```python
from build123d import *

# Parameters (mm, degrees)
SKETCH_1_R      = 1.75
SKETCH_1_W      = 12
SKETCH_1_H      = 4.5
EXTRUDE_1_DEPTH = 4.5
FILLET_1_R      = 12


with BuildPart() as part:
    # 草图1 → 凸台-拉伸1 (new body)
    with BuildSketch(Plane(origin=(0, 0, 0), x_dir=(1, 0, 0), z_dir=(0, 1, 0))):
        Polygon((29.444863729, 0), (14.722431864, 25.5), (-14.722431864, 25.5), (-29.444863729, 0), (-14.722431864, -25.5), (14.722431864, -25.5), align=None)
        Circle(SKETCH_1_R, mode=Mode.SUBTRACT)
        Polygon((13.887495374, 14.946152423), (9.990381057, 12.696152423), (15.990381057, 2.303847577), (19.887495374, 4.553847577), align=None, mode=Mode.SUBTRACT)
        with Locations((0, 17.25)):
            Rectangle(SKETCH_1_W, SKETCH_1_H, mode=Mode.SUBTRACT)
        Polygon((19.887495374, -4.553847577), (15.990381057, -2.303847577), (9.990381057, -12.696152423), (13.887495374, -14.946152423), align=None, mode=Mode.SUBTRACT)
        with Locations((0, -17.25)):
            Rectangle(SKETCH_1_W, SKETCH_1_H, mode=Mode.SUBTRACT)
        Polygon((-13.887495374, -14.946152423), (-9.990381057, -12.696152423), (-15.990381057, -2.303847577), (-19.887495374, -4.553847577), align=None, mode=Mode.SUBTRACT)
        Polygon((-19.887495374, 4.553847577), (-15.990381057, 2.303847577), (-9.990381057, 12.696152423), (-13.887495374, 14.946152423), align=None, mode=Mode.SUBTRACT)
    extrude(amount=EXTRUDE_1_DEPTH)

    # 圆角1
    fillet_1_edges = [part.edges().sort_by_distance(p)[0] for p in [
        (14.722431864, 2.25, 25.5),
        (-14.722431864, 2.25, 25.5),
        (-29.444863729, 2.25, 0),
        (-14.722431864, 2.25, -25.5),
        (14.722431864, 2.25, -25.5),
        (29.444863729, 2.25, 0),
    ]]
    fillet(fillet_1_edges, radius=FILLET_1_R)


solid = part.part
```
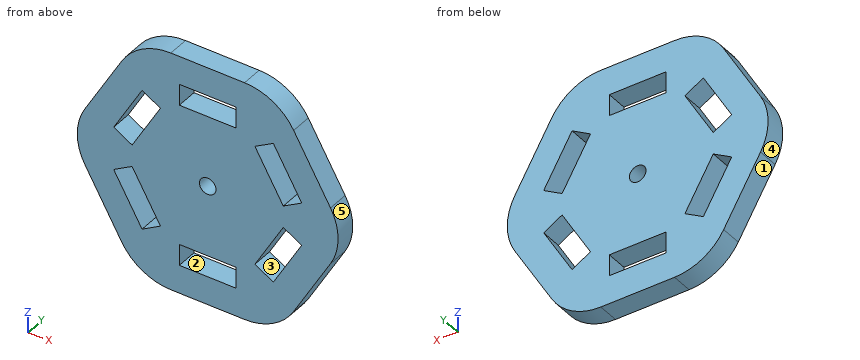
Check sheet for the modelled part. Datum: model origin and axes. Units: mm. Face numbers are marked on the shaded views. A direction names the side the tool comes from. Round coordinates to 2 decimals unless told otherwise and drop trailing zeros. Loops run counter-clockwise (first coordinate to the right, second up) from the corner with the lowest first, then second, coordinate; pieces in that order, holes last. Notation, with made-up numbers: (52.25, -13) - (111.25, -13) arc R23 cw to (111.25, 21) - close; hole circle Ø9 at (68.5, 69.25). An arc over 180 degrees is marked (long way). Write item = value, one per line. Start each with the question number.
Q1. Depth check by flat-ended pin: P1, Ø2, axis at y = 2.5, z = -16.5, coming from the -X side; P2, Ø3, axis at x = 0, z = 0, coming from the +Y side; P3, Ø2, axis at x = 20, y = 3, coming from the -Z side. Enter the tip coordinate at first touch or a pass-through.
Q2. Section check A-A (z = 0). Record the boundary of the cut face in (x, y).
Q3. Section check D-D (x = 15). Record the boundary of the cut face in (y, z).
Q4. Section check B-B (x = 0). Record the boundary of the cut face in (y, z).
Q5. Release check for a two-part mould opening along X. For the marked faces 3, 4 and 5 record: pulls with the +X half, pulls with the -X half, needs draft (parallel to the pull), parting line crosses it, or undercut.
Q6. Thickness scan on L1, parallel to Z at x = 0, y = 1.4; L2, parallel to Z at x = 4.5, y = 0.6; L3, parallel to X at y = 3.3, z = 0. Record the ranges inside material, lowest first.
Q7. Access from +Z, -Z, +X, -X, +Y, -Y to the whole of each face (thin tool, end or side, straight path). Record for the marked faces 1 and 2.
Q8. Section check C-C (z = 11). Record the boundary of the cut face in (x, y), plus the area to 3 significant figures.
Derived:
q1.P1 = -20.5
q1.P2 = through
q1.P3 = -18.09
q2.outline = (-27.59, 0) - (-1.75, 0) - (-1.75, 4.5) - (-27.59, 4.5) - close; (1.75, 0) - (27.59, 0) - (27.59, 4.5) - (1.75, 4.5) - close
q3.outline = (0, -23.1) - (4.5, -23.1) - (4.5, -13.02) - (0, -13.02) - close; (0, -4.02) - (4.5, -4.02) - (4.5, 4.02) - (0, 4.02) - close; (0, 13.02) - (4.5, 13.02) - (4.5, 23.1) - (0, 23.1) - close
q4.outline = (0, -25.5) - (4.5, -25.5) - (4.5, -19.5) - (0, -19.5) - close; (0, -15) - (4.5, -15) - (4.5, -1.75) - (0, -1.75) - close; (0, 1.75) - (4.5, 1.75) - (4.5, 15) - (0, 15) - close; (0, 19.5) - (4.5, 19.5) - (4.5, 25.5) - (0, 25.5) - close
q5.face_3 = undercut
q5.face_4 = pulls with the -X half
q5.face_5 = pulls with the +X half
q6.L1 = -25.5 to -19.5, -15 to -1.75, 1.75 to 15, 19.5 to 25.5
q6.L2 = -25.5 to -19.5, -15 to 15, 19.5 to 25.5
q6.L3 = -27.59 to -1.75, 1.75 to 27.59
q7.face_1 = -Z, -X, +Y, -Y
q7.face_2 = +Y, -Y
q8.outline = (-23.09, 0) - (-16.17, 0) - (-16.17, 4.5) - (-23.09, 4.5) - close; (-10.97, 0) - (10.97, 0) - (10.97, 4.5) - (-10.97, 4.5) - close; (16.17, 0) - (23.09, 0) - (23.09, 4.5) - (16.17, 4.5) - close
q8.area = 161 mm^2
